Check sheet for the drawn part. Datum: minimum x, y, z corner. Units: mm. A direction names the side the tool comes from. Coordinates: 2 decimals unless noted, no trailing zeros. Write each loop counter-clockwise with the first axis right and the second up, starting at its lowest first coordinate (ties: lowest second). Pieces come first, ordered by that corner, then holes. Notation, with made-up numbers: M -1,50.5 L 27,50.5 A11 cw 27,59.5 Z; hole C -34,83 d9. An arc over 180 degrees is marked long. Answer as CSV lines item,"result".
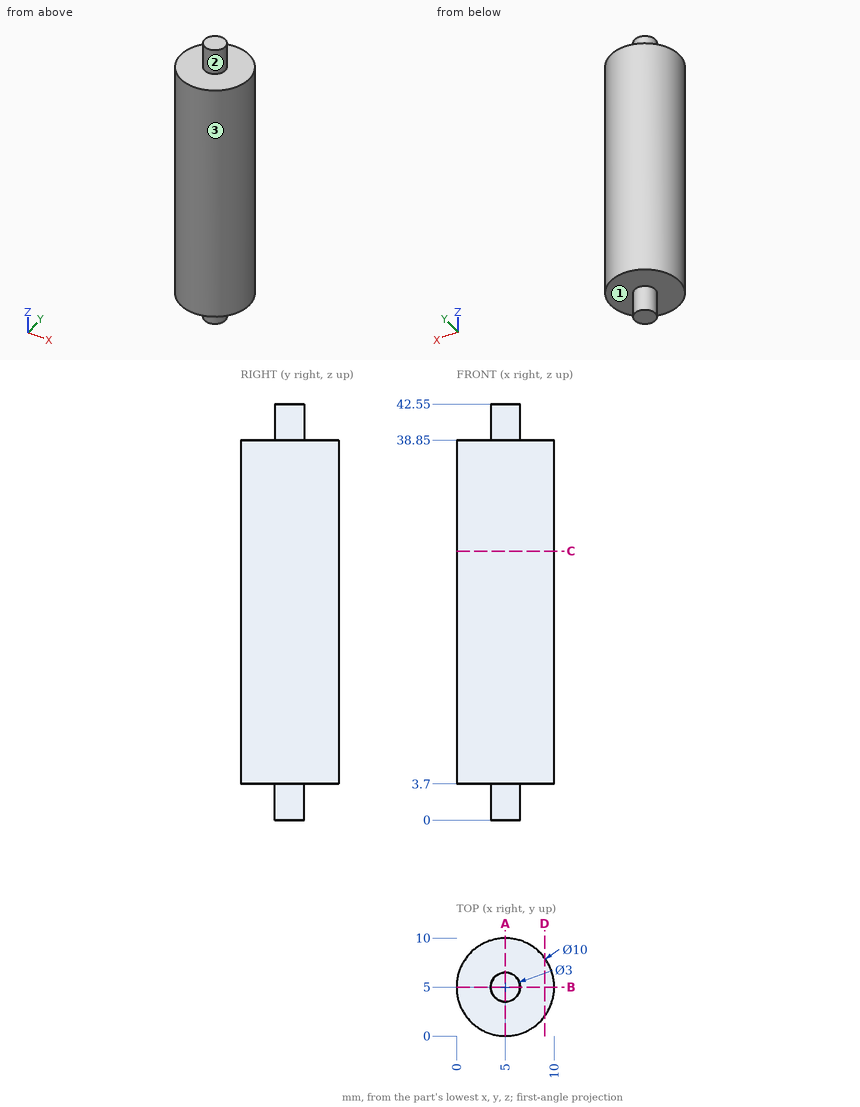
1) Depth check by flat-ended pin: P1, Ø2, axis at x = 3, y = 8.5, coming from the +Z side; P2, Ø2, axis at x = 7.5, y = 7.5, coming from the -Z side; P3, Ø4, axis at x = 3.5, y = 2, coming from the -Z side. Enter the tip coordinate at first touch or a pass-through.
Answer key:
P1,"stops at z = 38.85"
P2,"stops at z = 3.7"
P3,"stops at z = 0"
2) Thickness scan on line 1 along Z through (x, y) = (2, 4.75); line 2 along Y through (x, z) = (2, 8.5); line 3 along Y through (x, z) = (3.5, 37.5). Record the ranges inside material, lowest first.
Answer key:
line 1,"z = 3.7 to 38.85"
line 2,"y = 1 to 9"
line 3,"y = 0.23 to 9.77"
3) Section check A-A, the plane x = 5. Record the boundary of the cut face in (y, z).
Answer key:
outline,"M 0,3.7 L 3.5,3.7 L 3.5,0 L 6.5,0 L 6.5,3.7 L 10,3.7 L 10,38.85 L 6.5,38.85 L 6.5,42.55 L 3.5,42.55 L 3.5,38.85 L 0,38.85 Z"
4) Section check D-D, the plane x = 9. Record the boundary of the cut face in (y, z).
Answer key:
outline,"M 2,3.7 L 8,3.7 L 8,38.85 L 2,38.85 Z"
5) Tool access check on the marked faces 1, 2 and 3. Record the directions out of +Z, -Z, +X, -X, +Y, -Y that give a thin tool (end or side, any length) a straight path to the whole face; none if there is none.
Answer key:
face 1,"-Z"
face 2,"+Z"
face 3,"+Z, -Z"
6) Section check C-C, the plane z = 27.5. Record the boundary of the cut face in (x, y), plus the area to 3 significant figures.
Answer key:
outline,"C 5,5 d10"
area,"78.5 mm2"
